Part model, mm, in its own coordinate system. Round coordinates to 2 decimals unless told otherwise and drop trailing zeros. Order: outer loops, then holes, each group sorted by start corner. A loop starts at its lowest first (then second) coordinate and runs counter-clockwise, first axis right, second up. Notation, with made-up numbers: (-9.5, 53) - (7.5, 53) arc R19 ccw to (7.5, 76) - close; hole circle Ø10 at (73, 79.5). An arc over 180 degrees is marked (long way). Return JSON: item names as keys, results as strings. Group by question number.
Item 1: Drop flat-ended pins along their axis: pin 1 (10 mm diameter, centred on x = -13, z = 5.5, fed in from -Y); pin 2 (1.5 mm diameter, centred on x = 84.5, y = -6.5, fed in from +Z); pin 3 (2 mm diameter, centred on x = 36.5, y = -7.5, fed in from -Z); pin 4 (5.5 mm diameter, centred on x = -24, z = 0, fed in from -Y). Give the stop position or say it passes through.
Item 2: Probe probe 1 along X at (y, z) = (-8.2, 0); probe 2 along Y at (x, z) = (-11, 0). List the from-to ranges inside material, lowest first.
Item 3: Saw through at D-D on x = 52.5. List the corners of the cut face in (y, z).
Item 4: Two-plate mould, pull along Z, no slides. Class faces 1 (the face through (107, 8.2, 0)), 2 (the face through (-21.043, -8.669, -0.931)): released by +Z, released by -Z, zero draft, split by the parting line, or undercut.
Item 5: Saw through at B-B on z = 0. List the corners of the cut face in (x, y), and give its area (3 significant figures).
Item 6: Saw through at C-C on x = -25. List the corners of the cut face in (y, z), and give its area (3 significant figures).
Item 7: Saw through at A-A on y = 0. List the corners of the cut face in (x, z), and give its area (3 significant figures).
```python
from build123d import *

# Parameters (mm, degrees)
SKETCH_1_R          = 10
SKETCH_1_R_2        = 8
EXTRUDE_1_DEPTH     = 107
SKETCH_2_R          = 10
SKETCH_2_R_2        = 8
EXTRUDE_2_DEPTH     = 34
SKETCH_3_R          = 3
CUT_EXTRUDE_1_DEPTH = 15
SKETCH_4_R          = 3.1
CUT_EXTRUDE_2_DEPTH = 10


with BuildPart() as part:
    # 草图1 → 凸台-拉伸1 (new body)
    with BuildSketch(Plane(origin=(0, 0, 0), x_dir=(0, 0, -1), z_dir=(1, 0, 0))):
        Circle(SKETCH_1_R)
        Circle(SKETCH_1_R_2, mode=Mode.SUBTRACT)
    extrude(amount=EXTRUDE_1_DEPTH)

    # 草图2 → 凸台-拉伸2 (add)
    with BuildSketch(Plane.ZY):
        Circle(SKETCH_2_R)
        Circle(SKETCH_2_R_2, mode=Mode.SUBTRACT)
    extrude(amount=EXTRUDE_2_DEPTH)

    # 草图3 → 切除-拉伸1 (cut, symmetric)
    with BuildSketch(Plane(origin=(0, 0, 0), x_dir=(1, 0, 0), z_dir=(0, 1, 0))):
        with Locations((97, 0)):
            Circle(SKETCH_3_R)
    extrude(amount=CUT_EXTRUDE_1_DEPTH, both=True, mode=Mode.SUBTRACT)

    # 草图4 → 切除-拉伸2 (cut, symmetric)
    with BuildSketch(Plane(origin=(0, 0, 0), x_dir=(1, 0, 0), z_dir=(0, 1, 0))):
        with Locations((-24, 0)):
            Circle(SKETCH_4_R)
    extrude(amount=CUT_EXTRUDE_2_DEPTH, both=True, mode=Mode.SUBTRACT)


solid = part.part
```
Filled in:
{
 "1": {"pin 1": "stops at y = -9.99", "pin 2": "stops at z = 8.18", "pin 3": "stops at z = -7.6", "pin 4": "passes through"},
 "2": {"probe 1": "x = -34 to -27.1, -20.9 to 94, 100 to 107", "probe 2": "y = -10 to -8, 8 to 10"},
 "3": {"outline": "circle Ø20 at (0, 0); hole circle Ø16 at (0, 0)"},
 "4": {"face 1": "zero draft", "face 2": "undercut"},
 "5": {"outline": "(-34, -10) - (-27.1, -10) - (-27.1, -8) - (-34, -8) - close; (-34, 8) - (-27.1, 8) - (-27.1, 10) - (-34, 10) - close; (-20.9, -10) - (94, -10) - (94, -8) - (-20.9, -8) - close; (-20.9, 8) - (94, 8) - (94, 10) - (-20.9, 10) - close; (100, -10) - (107, -10) - (107, -8) - (100, -8) - close; (100, 8) - (107, 8) - (107, 10) - (100, 10) - close", "area": "515 mm^2"},
 "6": {"outline": "(-9.56, -2.93) arc R10 ccw to (9.56, -2.93) - (7.44, -2.93) arc R8 cw to (-7.44, -2.93) - close; (-9.56, 2.93) - (-7.44, 2.93) arc R8 cw to (7.44, 2.93) - (9.56, 2.93) arc R10 ccw to start", "area": "89.2 mm^2"},
 "7": {"outline": "(-34, -10) - (107, -10) - (107, -8) - (-34, -8) - close; (-34, 8) - (107, 8) - (107, 10) - (-34, 10) - close", "area": "564 mm^2"}
}
